The listing builds one solid part. Answer for the finished solid, in the listing's coordinates (mm). A direction names the side the tool comes from. Give positions to 0.01 mm unless a question says otherwise; leave off trailing zeros. Write each loop counter-clockwise with the first axis right and the second up, starting at its lowest first coordinate (ties: lowest second). Pieces come first, ordered by that corner, then holes.
```python
from build123d import *

# Parameters (mm, degrees)
BOSS_EXTRUDE3_DEPTH = 20
CUT_EXTRUDE3_DEPTH  = 20
BOSS_EXTRUDE4_DEPTH = 20
SKETCH5_W           = 10
SKETCH5_H           = 5
EXTRUDE_THIN1_DEPTH = 20
FILLET1_R           = 10
FILLET2_R           = 10
SKETCH6_R           = 6
CUT_EXTRUDE5_DEPTH  = 98.5
SKETCH7_W           = 25.027670854
SKETCH7_H           = 6.25
SKETCH7_W_2         = 25.066409398
CUT_EXTRUDE6_DEPTH  = 80.207653836
SKETCH8_R           = 6.011095122
BOSS_EXTRUDE6_DEPTH = 5
CUT_EXTRUDE9_DEPTH  = 35


with BuildPart() as part:
    # Sketch1 → Boss-Extrude3 (new body)
    with BuildSketch(Plane(origin=(0, 0, 0), x_dir=(0, 0, -1), z_dir=(1, 0, 0))):
        with BuildLine():
            Line((0, -17.661005955), (0, -97.661005955))
            Line((0, -97.661005955), (10, -97.661005955))
            Line((10, -97.661005955), (10, -115.161005955))
            Line((10, -115.161005955), (45, -115.161005955))
            ThreePointArc((45, -115.161005955), (79.207653836, -57.661005955), (45, -0.161005955))
            Line((45, -0.161005955), (10, -0.161005955))
            Line((10, -0.161005955), (10, -17.661005955))
            Line((10, -17.661005955), (0, -17.661005955))
        make_face()
    extrude(amount=BOSS_EXTRUDE3_DEPTH)

    # Sketch3 → Cut-Extrude3 (cut)
    with BuildSketch(Plane(origin=(20, 0, 0), x_dir=(0, 0, -1), z_dir=(1, 0, 0))):
        with BuildLine():
            Line((45, -17.661005955), (25, -17.661005955))
            Line((25, -17.661005955), (24.599094088, -97.970728365))
            Line((24.599094088, -97.970728365), (44.599094088, -97.970728365))
            ThreePointArc((44.599094088, -97.970728365), (64.519852612, -57.914310871), (45, -17.661005955))
        make_face()
    extrude(amount=-CUT_EXTRUDE3_DEPTH, mode=Mode.SUBTRACT)

    # Sketch4 → Boss-Extrude4 (add)
    with BuildSketch(Plane.XY):
        with BuildLine():
            Line((0, -17.661005955), (0, -32.661005955))
            Line((0, -32.661005955), (-20.64, -32.661005955))
            ThreePointArc((-20.64, -32.661005955), (-27.711067812, -29.732073767), (-30.64, -22.661005955))
            Line((-30.64, -22.661005955), (-40.64, -22.661005955))
            Line((-40.64, -22.661005955), (-40.64, -17.661005955))
            Line((-40.64, -17.661005955), (-80, -17.661005955))
            Line((-80, -17.661005955), (-79.933590602, -32.660858947))
            Line((-79.933590602, -32.660858947), (-54.933590602, -32.660858947))
            Line((-54.933590602, -32.660858947), (-54.933590602, -82.661005955))
            Line((-54.933590602, -82.661005955), (-80, -82.661005955))
            Line((-80, -82.661005955), (-80, -97.661005955))
            Line((-80, -97.661005955), (-40.64, -97.661005955))
            Line((-40.64, -97.661005955), (-40.64, -92.661005955))
            Line((-40.64, -92.661005955), (-30.64, -92.661005955))
            ThreePointArc((-30.64, -92.661005955), (-27.711067812, -85.589938143), (-20.64, -82.661005955))
            Line((-20.64, -82.661005955), (0, -82.661005955))
            Line((0, -82.661005955), (0, -97.661005955))
            Line((0, -97.661005955), (20, -97.661005955))
            Line((20, -97.661005955), (20, -17.661005955))
            Line((20, -17.661005955), (0, -17.661005955))
        make_face()
    extrude(amount=-BOSS_EXTRUDE4_DEPTH)

    # Sketch5 → Extrude-Thin1 (add)
    with BuildSketch(Plane.XY):
        with Locations((-35.64, -20.161005955)):
            Rectangle(SKETCH5_W, SKETCH5_H)
        with Locations((-35.64, -95.161005955)):
            Rectangle(SKETCH5_W, SKETCH5_H)
    extrude(amount=-EXTRUDE_THIN1_DEPTH)

    # Fillet1
    fillet1_edges = [part.edges().sort_by_distance(p)[0] for p in [
        (-30.64, -22.661005955, -10),
        (-30.64, -17.661005955, -10),
    ]]
    fillet(fillet1_edges, radius=FILLET1_R)

    # Fillet2
    fillet2_edges = [part.edges().sort_by_distance(p)[0] for p in [
        (-30.64, -97.661005955, -10),
        (-30.64, -92.661005955, -10),
    ]]
    fillet(fillet2_edges, radius=FILLET2_R)

    # Sketch6 → Cut-Extrude5 (cut, through all)
    with BuildSketch(Plane(origin=(0, -17.661005955, 0), x_dir=(1, 0, 0), z_dir=(0, 1, 0))):
        with Locations((-71.071972719, 11.735710253)):
            Circle(SKETCH6_R)
    extrude(amount=-CUT_EXTRUDE5_DEPTH, mode=Mode.SUBTRACT)

    # Sketch7 → Cut-Extrude6 (cut, through all)
    with BuildSketch(Plane.XY):
        with Locations((-67.447426029, -29.535858947)):
            Rectangle(SKETCH7_W, SKETCH7_H)
        with Locations((-67.466795301, -85.786005955)):
            Rectangle(SKETCH7_W_2, SKETCH7_H)
    extrude(amount=-CUT_EXTRUDE6_DEPTH, mode=Mode.SUBTRACT)

    # Sketch8 → Boss-Extrude6 (add)
    with BuildSketch(Plane(origin=(0, -17.661005955, 0), x_dir=(1, 0, 0), z_dir=(0, 1, 0))):
        with Locations((-71.071972719, 11.735710253)):
            Circle(SKETCH8_R)
    extrude(amount=BOSS_EXTRUDE6_DEPTH)

    # Sketch9 → Cut-Extrude9 (cut)
    with BuildSketch(Plane.XY):
        Polygon((-83.496027852, -22.661005955), (-54.933590602, -22.661005955), (-54.933590602, -92.661005955), (-84.905926437, -92.661005955), align=None)
    extrude(amount=-CUT_EXTRUDE9_DEPTH, mode=Mode.SUBTRACT)


solid = part.part
```
Item 1: A cutting plane is placed at B-B, the plane x = -56.5. Give the vertices of the cut face in (y, z), plus the area to 3 significant figures.
Conclusion:
outline: (-97.66, -20) - (-92.66, -20) - (-92.66, 0) - (-97.66, 0) - close; (-22.66, -20) - (-17.66, -20) - (-17.66, 0) - (-22.66, 0) - close
area: 200 mm2
Item 2: Determine the mould class of faces 5 (the face through (-65, -22.661, -10)), 6 (the face through (10, -115.161, -27)), 7 (the face through (10, -0.161, -28)), 8 (the face through (10, -97.971, -34)) for opening direction Y: pulls with the +Y half, pulls with the -Y half, needs draft (parallel to the pull), parting line crosses it, or undercut.
Conclusion:
face 5: undercut
face 6: pulls with the -Y half
face 7: pulls with the +Y half
face 8: undercut
Item 3: Which of the six approach directions +Z, -Z, +X, -X, +Y, -Y give full straight-line access (tool end or side, diameter ignored) to faces 1 (the face through (-71, -12.661, -12)), 2 (the face through (-26.691, -30.623, -9.86)), 3 (the face through (-54.934, -57, -10)), 4 (the face through (10, -106, -10))?
Conclusion:
face 1: +Z, -Z, -X, +Y
face 2: +Z, -Z, +Y
face 3: +Z, -Z, -X
face 4: +Z, +X, -X, -Y
Item 4: A cutting plane is placed at C-C, the plane y = -76.5. Give the vertices of the cut face in (x, z), plus the area to 3 significant figures.
Conclusion:
outline: (-54.93, -20) - (0, -20) - (0, -24.71) - (20, -24.71) - (20, 0) - (-54.93, 0) - close; (0, -76.44) - (20, -76.44) - (20, -60.89) - (0, -60.89) - close
area: 1,900 mm2
Item 5: A cutting plane is placed at D-D, the plane x = -67. Give the vertices of the cut face in (y, z).
Conclusion:
outline: (-97.66, -20) - (-92.66, -20) - (-92.66, -16.14) - (-97.66, -16.14) - close; (-97.66, -7.33) - (-92.66, -7.33) - (-92.66, 0) - (-97.66, 0) - close; (-22.66, -20) - (-17.66, -20) - (-17.66, -16.16) - (-12.66, -16.16) - (-12.66, -7.31) - (-17.66, -7.31) - (-17.66, 0) - (-22.66, 0) - (-22.66, -7.33) - (-17.66, -7.33) - (-17.66, -16.14) - (-22.66, -16.14) - close
Item 6: A cutting plane is placed at A-A, the plane z = -33. Give the vertices of the cut face in (x, y), plus the area to 3 significant figures.
Conclusion:
outline: (0, -115.16) - (20, -115.16) - (20, -97.97) - (0, -97.97) - close; (0, -17.66) - (20, -17.66) - (20, -0.16) - (0, -0.16) - close
area: 694 mm2
Item 7: Consider probe 1 along Y at (x, z) = (-60, -13.5); probe 2 along Y at (x, z) = (2, -27.5); probe 3 along X at (y, z) = (-28.5, -58). Determine where each line is inside the solid, lowest interval first.
Conclusion:
probe 1: y = -97.66 to -92.66, -22.66 to -17.66
probe 2: y = -115.16 to -97.97, -17.66 to -0.16
probe 3: x = 0 to 20
Item 8: Each of these flat-tipped pins is pushed along its axis until it touches: P1, Ø24, axis at x = -23.5, y = -61.5, coming from the -Z side; P2, Ø16, axis at y = -46.5, z = -10.5, coming from the -X side; P3, Ø1, axis at x = -10, z = -11, coming from the +Y side. Where does it stop, or does it pass through?
Conclusion:
P1: stops at z = -20
P2: stops at x = -54.93
P3: stops at y = -32.66
